Verification items for this drawing (mm, ordinates from the low corner). Coordinates: 2 decimals unless noted, no trailing zeros. Order: outer loops, then holes, each group sorted by start corner. A loop starts at its lowest first (then second) coordinate and runs counter-clockwise, first axis right, second up.
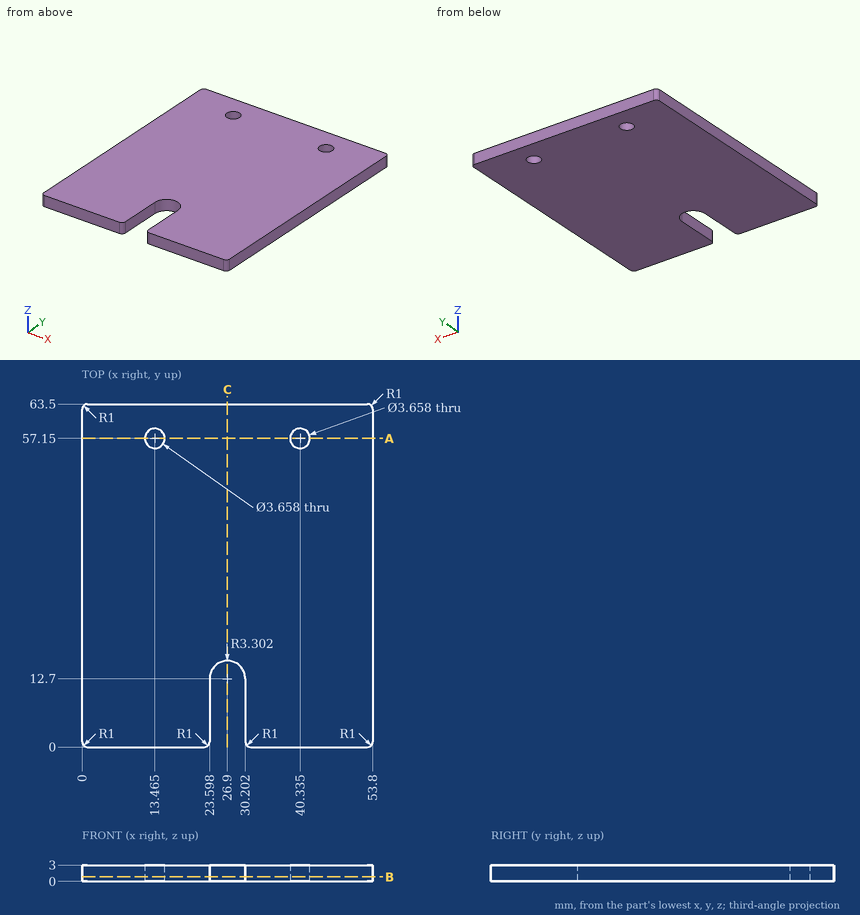
Item 1: Sectioned sample at B-B (z = 0.85). Give the number of separate pieces and of enclosed holes in the cut face, and give its area (3 significant figures).
Item 2: Sectioned sample at C-C (x = 26.9). Record the cut outline in (y, z).
Item 3: Thickness scan on line 1 along X through (y, z) = (3, 2.15); line 2 along X through (y, z) = (14.5, 2.2). Record the ranges inside material, lowest first.
Item 4: Sectioned sample at A-A (y = 57.15). Record the cut outline in (x, z).
Geometry check:
1. separate pieces: 1
1. enclosed holes: 2
1. area: 3,290 mm2
2. outline: (16, 0) - (63.5, 0) - (63.5, 3) - (16, 3) - close
3. line 1: x = 0 to 23.6, 30.2 to 53.8
3. line 2: x = 0 to 24.13, 29.67 to 53.8
4. outline: (0, 0) - (11.64, 0) - (11.64, 3) - (0, 3) - close; (15.29, 0) - (38.51, 0) - (38.51, 3) - (15.29, 3) - close; (42.16, 0) - (53.8, 0) - (53.8, 3) - (42.16, 3) - close
